Input: part model. Units: mm. Frame: model coordinates. A direction names the side the tool comes from. Give positions to 0.01 mm unless a question says otherwise; leave off trailing zeros. Loops run counter-clockwise (first coordinate to the right, second up) from the corner with the lowest first, then second, coordinate; pieces in that order, holes last. Notation, with made-up numbers: (6.25, 2.5) -> (10.25, 2.5) arc R14 ccw to (10.25, 12.5) -> close; hole circle Ø10 at (71, 16). An arc over 180 degrees is marked (long way). Answer in a Markdown table with one row per item. Add a question column.
Autodesk Inventor part; units mm, degrees
ref_plane "YZ Plane" through (0, 0, 0) normal (1, 0, 0) x (0, 1, 0)
ref_plane "XZ Plane" through (0, 0, 0) normal (0, 1, 0) x (-1, 0, 0)
ref_plane "XY Plane" through (0, 0, 0) normal (0, 0, 1) x (1, 0, 0)
sketch "Sketch1" plane through (0, 0, 0) normal (0, 0, 1) x (1, 0, 0)
  line L0 (-25.4, -12.7) -> (25.4, -12.7)
  line L1 (25.4, -12.7) -> (25.4, 12.7)
  line L2 (25.4, 12.7) -> (-25.4, 12.7)
  line L3 (-25.4, 12.7) -> (-25.4, -12.7)
  line L4 (-25.4, -12.7) -> (25.4, 12.7) construction
  line L5 (25.4, -12.7) -> (-25.4, 12.7) construction
  line L6 (-22.86, -10.16) -> (22.86, -10.16)
  line L7 (22.86, -10.16) -> (22.86, 10.16)
  line L8 (22.86, 10.16) -> (-22.86, 10.16)
  line L9 (-22.86, 10.16) -> (-22.86, -10.16)
  line L10 (-22.86, -10.16) -> (22.86, 10.16) construction
  line L11 (22.86, -10.16) -> (-22.86, 10.16) construction
  point P0 (0, 0)
  dimension "d0" = 50.8
  dimension "d1" = 25.4
  dimension "d2" = 45.72
  dimension "d3" = 20.32
extrude "Extrusion1" add sketch "Sketch1" along normal mid plane 381
sketch "Sketch2" plane through (25.4, -12.7, 190.5) normal (1, 0, 0) x (0, 0, -1)
  line L0 (381, 25.4) -> (0, 25.4)
  line L1 (0, 0) -> (0, 25.4)
  point P0 (190.5, 12.7)
  point P1 (12.7, 12.7)
  dimension "d6" = 12.7
  dimension "d7" = 12.7
hole "Hole1" at (25.4, 0, 177.8) direction (-1, 0, 0) diameter 4.1402 end through all
pattern_linear "Rectangular Pattern1" count 15 spacing 25.4 along (0, 0, -1) of "Hole1"
sketch "Sketch4" plane through (-25.4, -12.7, 190.5) normal (0, -1, 0) x (1, 0, 0)
  line L0 (0, 0) -> (50.8, 0)
  line L1 (50.8, -381) -> (50.8, 0)
  point P0 (25.4, -190.5)
  point P1 (38.1, -19.05)
  point P2 (12.7, -19.05)
  dimension "d38" = 25.4
  dimension "d39" = 19.05
  dimension "d40" = 12.7
hole "Hole4" at (12.7, -12.7, 171.45) at (-12.7, -12.7, 171.45) direction (0, 1, 0) diameter 4.1402 end through all
properties part number "Vertical_intake_frame"
1) Material intervals for line 1 along Z through (x, y) = (-12.7, 10.85); line 2 along Y through (x, z) = (-14, 108.5); line 3 along X through (y, z) = (9, -125.5), sorted ascending.
2) Reachability of faces 1 (the face through (-25.4, 0, -3)), 2 (the face through (0, 10.16, -3)) from +Z, -Z, +X, -X, +Y, -Y: full face, straight path, thin tool, end or side. Return the list, or none.
3) Pin query (flat end, axial travel): pin 1 (6.5 mm diameter, centred on x = -12.7, z = 171.45, fed in from -Y); pin 2 (2.5 mm diameter, centred on y = 0, z = 76.2, fed in from -X). Return the tip coordinate at first contact, or that it passes through.
4) Section A-A on z = 41.5. Output: boundary loops of the cut face in (x, y).
5) Pull-direction query (Y, two-part tool) for faces 3 (the face through (0, 12.7, -3)), 4 (the face through (-0.1, 10.4, 190.5)), 5 (the face through (22.86, 0, -3)), 6 (the face through (-22.86, 0, -3)); classes: +Y half, -Y half, draft (parallel to the pull), parting line (faces both ways), or undercut.
Working result:
| question | item | result |
|---|---|---|
| 1 | line 1 | z = -190.5 to 169.38, 173.52 to 190.5 |
| 1 | line 2 | y = -12.7 to -10.16, 10.16 to 12.7 |
| 1 | line 3 | x = -25.4 to -22.86, 22.86 to 25.4 |
| 2 | face 1 | +Z, -Z, -X, +Y, -Y |
| 2 | face 2 | +Z, -Z |
| 3 | pin 1 | stops at y = -12.7 |
| 3 | pin 2 | passes through |
| 4 | outline | (-25.4, -12.7) -> (25.4, -12.7) -> (25.4, 12.7) -> (-25.4, 12.7) -> close; hole (-22.86, -10.16) -> (22.86, -10.16) -> (22.86, 10.16) -> (-22.86, 10.16) -> close |
| 5 | face 3 | +Y half |
| 5 | face 4 | draft |
| 5 | face 5 | undercut |
| 5 | face 6 | undercut |
